Source: CAD feature listing. Evaluate the final solid. Frame: model axes, mm. A direction names the side the tool comes from. Give positions to 0.01 mm unless a question says otherwise; leave off trailing zeros. Loops run counter-clockwise (first coordinate to the right, second up) from the corner with the lowest first, then second, coordinate; pieces in that order, holes last.
from build123d import *

# Parameters (mm, degrees)
SALIENTE_EXTRUIR1_DEPTH = 60
CROQUIS2_W              = 80
CROQUIS2_H              = 8
SALIENTE_EXTRUIR2_DEPTH = 40
CROQUIS3_R              = 8
SALIENTE_EXTRUIR3_DEPTH = 8
MATRIZL1_COUNT          = 2
MATRIZL1_PITCH          = 74.62
CROQUIS5_R              = 8
CORTAR_EXTRUIR1_DEPTH   = 8
REDONDEO2_R             = 20
CORTAR_EXTRUIR2_DEPTH   = 16


with BuildPart() as part:
    # Croquis1 → Saliente-Extruir1 (new body)
    with BuildSketch(Plane.XY):
        Polygon((0, 0), (80, 0), (80, 20), (0, 40), align=None)
    extrude(amount=SALIENTE_EXTRUIR1_DEPTH)

    # Croquis2 → Saliente-Extruir2 (add)
    with BuildSketch(Plane.XY.offset(60)):
        with Locations((40, 4)):
            Rectangle(CROQUIS2_W, CROQUIS2_H)
    saliente_extruir2 = extrude(amount=SALIENTE_EXTRUIR2_DEPTH)

    # Simetría1: Saliente-Extruir2 across plane
    add(saliente_extruir2.mirror(Plane(origin=(0, 0, 30), x_dir=(1, 0, 0), z_dir=(0, 0, -1))))

    # Croquis3 → Saliente-Extruir3 (add)
    with BuildSketch(Plane(origin=(70.588235294, -17.647058824, 0), x_dir=(0, 0, -1), z_dir=(0.9701425, -0.242535625, 0))):
        with BuildLine():
            Line((-43.861166484, 66.797449732), (-60, 38.805700006))
            Line((-60, 38.805700006), (0, 38.805700006))
            Line((0, 38.805700006), (-16.138833516, 66.797449732))
            ThreePointArc((-16.138833516, 66.797449732), (-30, 74.805700006), (-43.861166484, 66.797449732))
        make_face()
        with Locations((-30, 58.805700006)):
            Circle(CROQUIS3_R, mode=Mode.SUBTRACT)
    saliente_extruir3 = extrude(amount=-SALIENTE_EXTRUIR3_DEPTH)

    # MatrizL1: Saliente-Extruir3 ×2
    with Locations(*[Vector(-0.9701425, 0.242535625, 0) * (i * MATRIZL1_PITCH) for i in range(1, MATRIZL1_COUNT)]):
        add(saliente_extruir3)

    # Croquis5 → Cortar-Extruir1 (cut)
    with BuildSketch(Plane(origin=(0, 8, 0), x_dir=(1, 0, 0), z_dir=(0, 1, 0))):
        with Locations((20, 20)):
            Circle(CROQUIS5_R)
        with Locations((60, 20)):
            Circle(CROQUIS5_R)
        with Locations((60, -80)):
            Circle(CROQUIS5_R)
        with Locations((20, -80)):
            Circle(CROQUIS5_R)
    extrude(amount=-CORTAR_EXTRUIR1_DEPTH, mode=Mode.SUBTRACT)

    # Redondeo2
    redondeo2_edges = [part.edges().sort_by_distance(p)[0] for p in [
        (0, 4, 100),
        (80, 4, 100),
        (0, 4, -40),
        (80, 4, -40),
    ]]
    fillet(redondeo2_edges, radius=REDONDEO2_R)

    # Croquis6 → Cortar-Extruir2 (cut)
    with BuildSketch(Plane(origin=(9.411764706, 37.647058824, 0), x_dir=(0.9701425, -0.242535625, 0), z_dir=(0.242535625, 0.9701425, 0))):
        Polygon((32.760687511, -10.370090848), (15.760687511, -20.185045424), (15.760687511, -39.814954576), (32.760687511, -49.629909152), (49.760687511, -39.814954576), (49.760687511, -20.185045424), align=None)
    extrude(amount=-CORTAR_EXTRUIR2_DEPTH, mode=Mode.SUBTRACT)


solid = part.part
1) Pull-direction query (Y, two-part tool) for faces 1 (the flat face through (7.129, 52.442, 7.956)), 2 (the cylindrical face through (74.297, 4.056, 93.986)), 3 (the flat face through (10.094, 48.044, 30.42)); classes: released by +Y, released by -Y, zero draft, split by the parting line, or undercut.
Checks:
face 1: released by +Y
face 2: zero draft
face 3: undercut
2) Cut plane B-B (x = 10.5). State how many separate pieces and enclosed holes the cut face has, and give its area (3 significant figures).
Checks:
separate pieces: 2
enclosed holes: 1
area: 3,410 mm2
3) Cut plane A-A (z = 78). Return loops of the section in (x, y), and give its area (3 significant figures).
Checks:
outline: (0, 0) - (12.25, 0) - (12.25, 8) - (0, 8) - close; (27.75, 0) - (52.25, 0) - (52.25, 8) - (27.75, 8) - close; (67.75, 0) - (80, 0) - (80, 8) - (67.75, 8) - close
area: 392 mm2
4) Reachability of faces 4 (the flat face through (80, 8, 31)), 5 (the flat face through (31, 21, 60)), 6 (the flat face through (55.774, 17.926, 30.137)) from +Z, -Z, +X, -X, +Y, -Y: full face, straight path, thin tool, end or side. Return the list, or none.
Checks:
face 4: +Z, -Z, +X, -Y
face 5: +Z, +X, -X, +Y
face 6: +Y
5) Ray query, probe 1 along X at (y, z) = (2, -20); probe 2 along Z at (x, y) = (20, 6); probe 3 along Y at (x, z) = (78.5, -18.5). Return the intervals inside material, ascending.
Checks:
probe 1: x = 0 to 12, 28 to 52, 68 to 80
probe 2: z = -40 to -28, -12 to 72, 88 to 100
probe 3: y = 0 to 8
6) Cut plane C-C (z = -23). Return loops of the section in (x, y), and give its area (3 significant figures).
Checks:
outline: (0.23, 0) - (12.58, 0) - (12.58, 8) - (0.23, 8) - close; (27.42, 0) - (52.58, 0) - (52.58, 8) - (27.42, 8) - close; (67.42, 0) - (79.77, 0) - (79.77, 8) - (67.42, 8) - close
area: 399 mm2
7) Contact query for flat-ended pins moving along their axis: P1, Ø12, axis at y = 25, z = 51, coming from the -X side; P2, Ø16, axis at y = 14.5, z = 13.5, coming from the +X side (3 decimals); P3, Ø2, axis at y = 33.5, z = 33.5, coming from the +X side; P4, Ø14.5, axis at x = 60, z = 80, coming from the -Y side. Output: stop coordinate, or through.
Checks:
P1: stops at x = 0
P2: stops at x = 80.625
P3: stops at x = 83.2
P4: passes through
8) Cut plane D-D (x = 44). Return loops of the section in (y, z).
Checks:
outline: (0, -40) - (8, -40) - (8, 0) - (29, 0) - (29, 12.04) - (12.51, 14.35) - (12.51, 45.65) - (29, 47.96) - (29, 60) - (8, 60) - (8, 100) - (0, 100) - close
